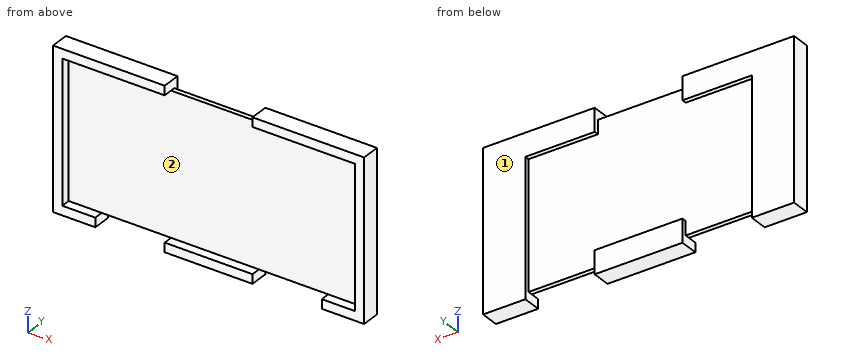
```python
from build123d import *

# Parameters (mm, degrees)
SKETCH_1_W          = 67.3
SKETCH_1_H          = 34.5
EXTRUDE_1_DEPTH     = 4
SKETCH_2_W          = 15
SKETCH_2_H          = 29.5
CUT_EXTRUDE_1_DEPTH = 1
SKETCH_3_W          = 63.3
SKETCH_3_H          = 30.5
CUT_EXTRUDE_2_DEPTH = 2
SKETCH_4_W          = 15
SKETCH_4_H          = 3
CUT_EXTRUDE_3_DEPTH = 2
SKETCH_6_W          = 19
SKETCH_6_H          = 29.5
CUT_EXTRUDE_5_DEPTH = 1
SKETCH_5_W          = 19
SKETCH_5_H          = 3
CUT_EXTRUDE_4_DEPTH = 2


with BuildPart() as part:
    # Эскиз1 → Бобышка-Вытянуть1 (new body)
    with BuildSketch(Plane(origin=(0, 0, 0), x_dir=(1, 0, 0), z_dir=(0, 1, 0))):
        Rectangle(SKETCH_1_W, SKETCH_1_H)
    extrude(amount=EXTRUDE_1_DEPTH)

    # Эскиз2 → Вырез-Вытянуть1 (cut)
    with BuildSketch(Plane(origin=(0, 4, 0), x_dir=(1, 0, 0), z_dir=(0, 1, 0))):
        with Locations((-17, 2.5)):
            Rectangle(SKETCH_2_W, SKETCH_2_H)
        with Locations((17, 2.5)):
            Rectangle(SKETCH_2_W, SKETCH_2_H)
    extrude(amount=-CUT_EXTRUDE_1_DEPTH, mode=Mode.SUBTRACT)

    # Эскиз3 → Вырез-Вытянуть2 (cut)
    with BuildSketch(Plane(origin=(0, 0, 0), x_dir=(-1, 0, 0), z_dir=(0, -1, 0))):
        Rectangle(SKETCH_3_W, SKETCH_3_H)
    extrude(amount=-CUT_EXTRUDE_2_DEPTH, mode=Mode.SUBTRACT)

    # Эскиз4 → Вырез-Вытянуть3 (cut)
    with BuildSketch(Plane(origin=(0, 0, -17.25), x_dir=(-1, 0, 0), z_dir=(0, 0, -1))):
        with Locations((-17, 1.5)):
            Rectangle(SKETCH_4_W, SKETCH_4_H)
        with Locations((17, 1.5)):
            Rectangle(SKETCH_4_W, SKETCH_4_H)
    extrude(amount=-CUT_EXTRUDE_3_DEPTH, mode=Mode.SUBTRACT)

    # Эскиз6 → Вырез-Вытянуть5 (cut)
    with BuildSketch(Plane(origin=(0, 4, 0), x_dir=(1, 0, 0), z_dir=(0, 1, 0))):
        with Locations((0, -2.5)):
            Rectangle(SKETCH_6_W, SKETCH_6_H)
    extrude(amount=-CUT_EXTRUDE_5_DEPTH, mode=Mode.SUBTRACT)

    # Эскиз5 → Вырез-Вытянуть4 (cut)
    with BuildSketch(Plane.XY.offset(17.25)):
        with Locations((0, 1.5)):
            Rectangle(SKETCH_5_W, SKETCH_5_H)
    extrude(amount=-CUT_EXTRUDE_4_DEPTH, mode=Mode.SUBTRACT)


solid = part.part
```
Here's how the part is built. I have some questions about the finished solid (model axes, mm). Face numbers are marked on the shaded views. Give positions to 0.01 mm unless a question says otherwise; leave off trailing zeros. Write each loop counter-clockwise with the first axis right and the second up, starting at its lowest first coordinate (ties: lowest second). Pieces come first, ordered by that corner, then holes.
(1) Will these pins go through, and if not, where does the flat tip stop? pin 1 (8 mm diameter, centred on x = 6, z = 13, fed in from -Y); pin 2 (1.6 mm diameter, centred on x = -19, y = 1.5, fed in from -Z); pin 3 (2 mm diameter, centred on x = 14, z = 2, fed in from +Y).
Output values:
pin 1: stops at y = 2
pin 2: stops at z = -15.25
pin 3: stops at y = 3
(2) Thinking about a two-plate mould opening in Z: for the marked faces 1 and 2, which applies, pulls with the +Z half, pulls with the -Z half, needs draft (parallel to the pull), parting line crosses it, or undercut?
Output values:
face 1: needs draft
face 2: undercut
(3) Imagine slicing it at C-C, the plane x = -13. Write out the boundary of the cut face in (y, z), and give its area (3 significant figures).
Output values:
outline: (0, 15.25) - (2, 15.25) - (2, -15.25) - (3, -15.25) - (3, 12.25) - (4, 12.25) - (4, 17.25) - (0, 17.25) - close
area: 41.5 mm2
(4) If I drill on L1, parallel to X at y = 1.85, z = -14; L2, parallel to X at y = 3.15, z = -10; L3, parallel to Z at x = -27, y = 1.7, over which ranges is the centre line in solid material (lowest first)?
Output values:
L1: x = -33.65 to -31.65, 31.65 to 33.65
L2: x = -33.65 to -24.5, 24.5 to 33.65
L3: z = -17.25 to -15.25, 15.25 to 17.25
(5) Imagine slicing it at B-B, the plane z = -0.5. Write out the boundary of the cut face in (x, y).
Output values:
outline: (-33.65, 0) - (-31.65, 0) - (-31.65, 2) - (31.65, 2) - (31.65, 0) - (33.65, 0) - (33.65, 4) - (24.5, 4) - (24.5, 3) - (-24.5, 3) - (-24.5, 4) - (-33.65, 4) - close
(6) Imagine slicing it at A-A, the plane x = -26.5. Write out the boundary of the cut face in (y, z).
Output values:
outline: (0, -17.25) - (4, -17.25) - (4, 17.25) - (0, 17.25) - (0, 15.25) - (2, 15.25) - (2, -15.25) - (0, -15.25) - close
